Could you check a few things on this model? Use its own coordinates, in mm. Give positions to 0.01 mm unless a question says otherwise; leave off trailing zeros. Loops run counter-clockwise (first coordinate to the right, second up) from the corner with the lowest first, then second, coordinate; pieces in that order, holes last. Notation, with made-up numbers: (-19, 58) - (-11, 58) arc R21 ccw to (-11, 72) - close; hole circle Ø4 at (-30, 25.25). An arc over 180 degrees is marked (long way). One line per item, written item: value. Start each with the question number.
Q1. If I drill on line 1 (Z direction, x = -67.25, y = -10) (3 decimals), over which ranges is the centre line in solid material (lowest first)? Write a range as from..to.
Q2. I want a section at B-B (z = 0). Please give me the cut outline in (x, y) (3 decimals), then the cut area to 3 significant figures.
Q3. I want a section at A-A (x = -61.5). Please give me the cut outline in (y, z) (3 decimals).
Q4. I'm going to push flat-ended pins straight in: P1, Ø3, axis at y = -10, z = -36, coming from the -X side; P2, Ø2, axis at x = 29, z = 23.5, coming from the +Y side. Where does each tip first touch, or does it pass through?
```python
from build123d import *

# Parameters (mm, degrees)
F0_W     = 140
F0_H     = 140
F1_DEPTH = 20
F3_DEPTH = 10
F4_DEPTH = 28.75


with BuildPart() as f1:
    # F0 (on Front) → F1 (new body)
    with BuildSketch(Plane.XZ):
        Rectangle(F0_W, F0_H)
    extrude(amount=F1_DEPTH)

    # F2 (on face) → F3 (cut)
    with BuildSketch(Plane(origin=(-70, 0, 0), x_dir=(0, -1, 0), z_dir=(-1, 0, 0))):
        with BuildLine():
            Line((6.825, 35.0000062), (13.175, 35.0000062))
            ThreePointArc((13.175, 35.0000062), (10, 38.1750062), (6.825, 35.0000062))
        make_face()
        with BuildLine():
            ThreePointArc((6.825, 35.0000062), (10, 31.8250062), (13.175, 35.0000062))
            Line((13.175, 35.0000062), (6.825, 35.0000062))
        make_face()
        with BuildLine():
            Line((6.825, 0), (13.175, 0))
            ThreePointArc((13.175, 0), (10, 3.175), (6.825, 0))
        make_face()
        with BuildLine():
            ThreePointArc((6.825, 0), (10, -3.175), (13.175, 0))
            Line((13.175, 0), (6.825, 0))
        make_face()
        with BuildLine():
            Line((6.825, -35.0000062), (13.175, -35.0000062))
            ThreePointArc((13.175, -35.0000062), (10, -31.8250062), (6.825, -35.0000062))
        make_face()
        with BuildLine():
            ThreePointArc((6.825, -35.0000062), (10, -38.1750062), (13.175, -35.0000062))
            Line((13.175, -35.0000062), (6.825, -35.0000062))
        make_face()
    extrude(amount=-F3_DEPTH, mode=Mode.SUBTRACT)

    # F4 (cut): a face of the model
    f4_faces = [f1.faces().sort_by_distance(p)[0] for p in [
        (70, -10, 0),
    ]]
    extrude(f4_faces, amount=-F4_DEPTH, mode=Mode.SUBTRACT)


solid = f1.part
```
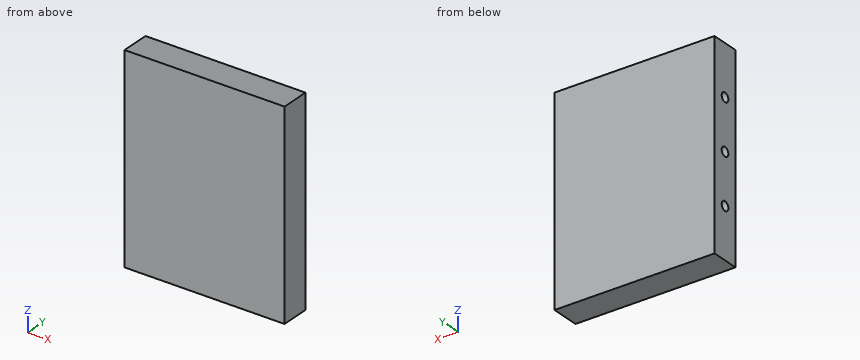
Worked answers:
1. line 1: z = -70..-38.175, -31.825..-3.175, 3.175..31.825, 38.175..70
2. outline: (-70, -20) - (41.25, -20) - (41.25, 0) - (-70, 0) - (-70, -6.825) - (-60, -6.825) - (-60, -13.175) - (-70, -13.175) - close
2. area: 2,160 mm²
3. outline: (-20, -70) - (0, -70) - (0, 70) - (-20, 70) - close; hole circle Ø6.35 at (-10, -35); hole circle Ø6.35 at (-10, 0); hole circle Ø6.35 at (-10, 35)
4. P1: stops at x = -60
4. P2: stops at y = 0
